Part model, mm, in its own coordinate system. A direction names the side the tool comes from. Give positions to 0.01 mm unless a question says otherwise; leave off trailing zeros. Write each loop counter-clockwise with the first axis right and the second up, starting at its lowest first coordinate (ties: lowest second). Pieces come first, ordered by that corner, then holes.
Autodesk Inventor part; units mm, degrees
ref_plane "HUELSE3_1_XY" through (11.8, 0, -12.5) normal (1, 0, 0) x (0, 0, -1)
ref_plane "HUELSE3_1_YZ" through (11.8, 0, -12.5) normal (0, 0, -1) x (0, 1, 0)
ref_plane "HUELSE3_1_ZX" through (11.8, 0, -12.5) normal (0, 1, 0) x (1, 0, 0)
sketch "Sketch_2" plane through (13, 0, 0) normal (1, 0, 0) x (0, 0, -1)
  line L0 (-29, -12) -> (-28, -13)
  line L1 (-28, -13) -> (28, -13)
  line L2 (28, -13) -> (29, -12)
  line L3 (29, -12) -> (29, 12)
  line L4 (29, 12) -> (28, 13)
  line L5 (28, 13) -> (-28, 13)
  line L6 (-28, 13) -> (-29, 12)
  line L7 (-29, 12) -> (-29, -12)
sketch "Sketch_3" plane through (0, 0, 0) normal (0, 1, 0) x (1, 0, 0)
  line L0 (13, 20.5) -> (-142, 20.5)
  line L1 (-142, 20.5) -> (-142, 24.5)
  line L2 (-142, 24.5) -> (-141, 25.5)
  line L3 (-141, 25.5) -> (13, 25.5)
  line L4 (13, 25.5) -> (13, 20.5)
  line L5 (13, 20.5) -> (-142, 20.5)
sketch "Sketch_4" plane through (0, 0, 0) normal (0, 1, 0) x (1, 0, 0)
  line L0 (13, -20.5) -> (-142, -20.5)
  line L1 (-142, -20.5) -> (-142, -16.5)
  line L2 (-142, -16.5) -> (-141, -15.5)
  line L3 (-141, -15.5) -> (13, -15.5)
  line L4 (13, -15.5) -> (13, -20.5)
  line L5 (13, -20.5) -> (-142, -20.5)
extrude "Extrusion1" add sketch "Sketch_2" against normal blind 10
sketch "Sketch_8" plane through (0, 10, 0) normal (0, 1, 0) x (1, 0, 0)
  line L0 (13, 10) -> (3, 10)
  line L1 (3, 10) -> (3, 12)
  line L2 (3, 12) -> (3.379, 11.621)
  line L3 (3.379, 11.621) -> (12.621, 11.621)
  line L4 (12.621, 11.621) -> (13, 12)
  line L5 (13, 12) -> (13, 10)
  line L6 (13, 10) -> (3, 10)
revolve "Revolution1" cut sketch "Sketch_8" angle 360 about axis through (13, 10, -10) along (-1, 0, 0)
thread "Thread1"
sketch "Sketch_9" plane through (0, 10, 0) normal (0, 1, 0) x (1, 0, 0)
  line L0 (13, -10) -> (3, -10)
  line L1 (3, -10) -> (3, -8)
  line L2 (3, -8) -> (3.379, -8.379)
  line L3 (3.379, -8.379) -> (12.621, -8.379)
  line L4 (12.621, -8.379) -> (13, -8)
  line L5 (13, -8) -> (13, -10)
  line L6 (13, -10) -> (3, -10)
revolve "Revolution2" cut sketch "Sketch_9" angle 360 about axis through (13, 10, 10) along (-1, 0, 0)
thread "Thread2"
sketch "Sketch_12" plane through (0, -10, 0) normal (0, 1, 0) x (1, 0, 0)
  line L0 (13, 10) -> (3, 10)
  line L1 (3, 10) -> (3, 12)
  line L2 (3, 12) -> (3.379, 11.621)
  line L3 (3.379, 11.621) -> (12.621, 11.621)
  line L4 (12.621, 11.621) -> (13, 12)
  line L5 (13, 12) -> (13, 10)
  line L6 (13, 10) -> (3, 10)
revolve "Revolution3" cut sketch "Sketch_12" angle 360 about axis through (13, -10, -10) along (-1, 0, 0)
thread "Thread3"
sketch "Sketch_13" plane through (0, -10, 0) normal (0, 1, 0) x (1, 0, 0)
  line L0 (13, -10) -> (3, -10)
  line L1 (3, -10) -> (3, -8)
  line L2 (3, -8) -> (3.379, -8.379)
  line L3 (3.379, -8.379) -> (12.621, -8.379)
  line L4 (12.621, -8.379) -> (13, -8)
  line L5 (13, -8) -> (13, -10)
  line L6 (13, -10) -> (3, -10)
revolve "Revolution4" cut sketch "Sketch_13" angle 360 about axis through (13, -10, 10) along (-1, 0, 0)
thread "Thread4"
sketch "Skizze_3" plane through (0, 0, 0) normal (0, 0, 1) x (1, 0, 0)
  line L0 (3, 0) -> (-117.4, 0)
  line L1 (-117.4, 0) -> (-117.4, 6)
  line L2 (-117.4, 6) -> (-111.4, 6)
  line L3 (-111.4, 6) -> (-111.4, 3)
  line L4 (-111.4, 3) -> (3, 3)
  line L5 (3, 3) -> (3, 0)
  line L6 (3, 0) -> (-117.4, 0)
revolve "Revolution5" add sketch "Skizze_3" angle 360 about axis through (3, 0, 0) along (-1, 0, 0)
sketch "Sketch_17" plane through (0, 0, 0) normal (1, 0, 0) x (0, 1, 0)
  line L0 (-10, 7.5) -> (-10, -7.5)
  line L1 (-10, -7.5) -> (10, -7.5)
  line L2 (10, -7.5) -> (10, 7.5)
  line L3 (10, 7.5) -> (-10, 7.5)
  line L4 (-5, 2.75) -> (-5, -2.75)
  line L5 (-5, -2.75) -> (5, -2.75)
  line L6 (5, -2.75) -> (5, 2.75)
  line L7 (5, 2.75) -> (-5, 2.75)
extrude "Extrusion2" cut sketch "Sketch_17" along normal blind 3
sketch "Sketch10" plane through (13, 0, 0) normal (1, 0, 0) x (0, 0, -1)
  point P0 (12.5, 0)
hole "Hole1" at (13, 0, -12.5) direction (-1, 0, 0) diameter 5 depth 1.2 tip angle 120
sketch "Sketch11" plane through (13, 0, 0) normal (1, 0, 0) x (0, 0, -1)
  point P0 (-12.5, 0)
hole "Hole2" at (13, 0, 12.5) direction (-1, 0, 0) diameter 5 depth 1.2 tip angle 120
sketch "Sketch12" plane through (13, 13, 28) normal (0, 1, 0) x (1, 0, 0)
  point P0 (-5, 48.5)
hole "Hole3" at (8, 13, -20.5) direction (0, -1, 0) diameter 3.242 depth 13 countersink diameter 4 countersink angle 90
sketch "Sketch13" plane through (13, 13, 28) normal (0, 1, 0) x (1, 0, 0)
  point P0 (-5, 7.5)
hole "Hole4" at (8, 13, 20.5) direction (0, -1, 0) diameter 3.242 depth 13 countersink diameter 4 countersink angle 90
revolve "Revolution6" add sketch "Sketch_4" angle 360 about axis through (13, 0, 20.5) along (1, 0, 0)
revolve "Revolution7" add sketch "Sketch_3" angle 360 about axis through (13, 0, -20.5) along (1, 0, 0)
sketch "Sketch_20" plane through (13, 0, 0) normal (1, 0, 0) x (0, 0, -1)
  arc A0 (-1.6342, -0.5011) -> (-1.2511, -1.1647) centre (-1.364, -0.7875) ccw
  arc A1 (-0.3831, -1.6659) -> (-1.2511, -1.1647) centre (-1.0536, -1.8249) ccw
  arc A2 (-0.3831, -1.6659) -> (0.3831, -1.6659) centre (0, -1.575) ccw
  arc A3 (1.2511, -1.1647) -> (0.3831, -1.6659) centre (1.0536, -1.8249) ccw
  arc A4 (1.2511, -1.1647) -> (1.6342, -0.5011) centre (1.364, -0.7875) ccw
  arc A5 (1.6342, 0.5011) -> (1.6342, -0.5011) centre (2.1072, 0) ccw
  arc A6 (1.6342, 0.5011) -> (1.2511, 1.1647) centre (1.364, 0.7875) ccw
  arc A7 (0.3831, 1.6659) -> (1.2511, 1.1647) centre (1.0536, 1.8249) ccw
  arc A8 (0.3831, 1.6659) -> (-0.3831, 1.6659) centre (0, 1.575) ccw
  arc A9 (-1.2511, 1.1647) -> (-0.3831, 1.6659) centre (-1.0536, 1.8249) ccw
  arc A10 (-1.2511, 1.1647) -> (-1.6342, 0.5011) centre (-1.364, 0.7875) ccw
  arc A11 (-1.6342, -0.5011) -> (-1.6342, 0.5011) centre (-2.1072, 0) ccw
extrude "Extrusion3" cut sketch "Sketch_20" against normal blind 2
sketch "Pattern_2_SKETCH_1" plane through (13, 0, 0) normal (1, 0, 0) x (0, 0, -1)
  arc A0 (18.8658, -0.5011) -> (19.2489, -1.1647) centre (19.136, -0.7875) ccw
  arc A1 (20.1169, -1.6659) -> (19.2489, -1.1647) centre (19.4464, -1.8249) ccw
  arc A2 (20.1169, -1.6659) -> (20.8831, -1.6659) centre (20.5, -1.575) ccw
  arc A3 (21.7511, -1.1647) -> (20.8831, -1.6659) centre (21.5536, -1.8249) ccw
  arc A4 (21.7511, -1.1647) -> (22.1342, -0.5011) centre (21.864, -0.7875) ccw
  arc A5 (22.1342, 0.5011) -> (22.1342, -0.5011) centre (22.6072, 0) ccw
  arc A6 (22.1342, 0.5011) -> (21.7511, 1.1647) centre (21.864, 0.7875) ccw
  arc A7 (20.8831, 1.6659) -> (21.7511, 1.1647) centre (21.5536, 1.8249) ccw
  arc A8 (20.8831, 1.6659) -> (20.1169, 1.6659) centre (20.5, 1.575) ccw
  arc A9 (19.2489, 1.1647) -> (20.1169, 1.6659) centre (19.4464, 1.8249) ccw
  arc A10 (19.2489, 1.1647) -> (18.8658, 0.5011) centre (19.136, 0.7875) ccw
  arc A11 (18.8658, -0.5011) -> (18.8658, 0.5011) centre (18.3928, 0) ccw
sketch "Pattern_2_SKETCH_2" plane through (13, 0, 0) normal (1, 0, 0) x (0, 0, -1)
  arc A0 (-22.1342, -0.5011) -> (-21.7511, -1.1647) centre (-21.864, -0.7875) ccw
  arc A1 (-20.8831, -1.6659) -> (-21.7511, -1.1647) centre (-21.5536, -1.8249) ccw
  arc A2 (-20.8831, -1.6659) -> (-20.1169, -1.6659) centre (-20.5, -1.575) ccw
  arc A3 (-19.2489, -1.1647) -> (-20.1169, -1.6659) centre (-19.4464, -1.8249) ccw
  arc A4 (-19.2489, -1.1647) -> (-18.8658, -0.5011) centre (-19.136, -0.7875) ccw
  arc A5 (-18.8658, 0.5011) -> (-18.8658, -0.5011) centre (-18.3928, 0) ccw
  arc A6 (-18.8658, 0.5011) -> (-19.2489, 1.1647) centre (-19.136, 0.7875) ccw
  arc A7 (-20.1169, 1.6659) -> (-19.2489, 1.1647) centre (-19.4464, 1.8249) ccw
  arc A8 (-20.1169, 1.6659) -> (-20.8831, 1.6659) centre (-20.5, 1.575) ccw
  arc A9 (-21.7511, 1.1647) -> (-20.8831, 1.6659) centre (-21.5536, 1.8249) ccw
  arc A10 (-21.7511, 1.1647) -> (-22.1342, 0.5011) centre (-21.864, 0.7875) ccw
  arc A11 (-22.1342, -0.5011) -> (-22.1342, 0.5011) centre (-22.6072, 0) ccw
extrude "Extrusion4" cut sketch "Pattern_2_SKETCH_1" against normal blind 2
extrude "Extrusion5" cut sketch "Pattern_2_SKETCH_2" against normal blind 2
sketch "Sketch_22" plane through (0, 0, 0) normal (0, 1, 0) x (1, 0, 0)
  line L0 (13, 0) -> (12.6, 0)
  line L1 (12.6, 0) -> (12.6, 3)
  arc A0 (12.6, 3) -> (12.1, 3.5) centre (12.1, 3) ccw
  line L2 (12.1, 3.5) -> (9.5, 3.5)
  line L3 (9.5, 3.5) -> (9.5, 4)
  line L4 (9.5, 4) -> (13, 4)
  line L5 (13, 4) -> (13, 0)
  line L6 (13, 0) -> (12.6, 0)
revolve "Revolution8" cut sketch "Sketch_22" angle 360 about axis through (13, 0, 0) along (-1, 0, 0)
sketch "Pattern_3_SKETCH_1" plane through (0, 0, 20.5) normal (0, 1, 0) x (1, 0, 0)
  line L0 (13, 0) -> (12.6, 0)
  line L1 (12.6, 0) -> (12.6, 3)
  arc A0 (12.6, 3) -> (12.1, 3.5) centre (12.1, 3) ccw
  line L2 (12.1, 3.5) -> (9.5, 3.5)
  line L3 (9.5, 3.5) -> (9.5, 4)
  line L4 (9.5, 4) -> (13, 4)
  line L5 (13, 4) -> (13, 0)
  line L6 (13, 0) -> (12.6, 0)
sketch "Pattern_3_SKETCH_2" plane through (0, 0, -20.5) normal (0, 1, 0) x (1, 0, 0)
  line L0 (13, 0) -> (12.6, 0)
  line L1 (12.6, 0) -> (12.6, 3)
  arc A0 (12.6, 3) -> (12.1, 3.5) centre (12.1, 3) ccw
  line L2 (12.1, 3.5) -> (9.5, 3.5)
  line L3 (9.5, 3.5) -> (9.5, 4)
  line L4 (9.5, 4) -> (13, 4)
  line L5 (13, 4) -> (13, 0)
  line L6 (13, 0) -> (12.6, 0)
revolve "Revolution9" cut sketch "Pattern_3_SKETCH_1" angle 360 about axis through (13, 0, 20.5) along (-1, 0, 0)
revolve "Revolution10" cut sketch "Pattern_3_SKETCH_2" angle 360 about axis through (13, 0, -20.5) along (-1, 0, 0)
ref_plane "HUELSE3_1_XY" through (11.8, 0, -12.5) normal (1, 0, 0) x (0, 0, -1)
ref_plane "HUELSE3_1_YZ" through (11.8, 0, -12.5) normal (0, 0, -1) x (0, 1, 0)
ref_plane "HUELSE3_1_ZX" through (11.8, 0, -12.5) normal (0, 1, 0) x (1, 0, 0)
ref_plane "HUELSE3_2_XY" through (11.8, 0, 12.5) normal (1, 0, 0) x (0, 0, -1)
ref_plane "HUELSE3_2_YZ" through (11.8, 0, 12.5) normal (0, 0, -1) x (0, 1, 0)
ref_plane "HUELSE3_2_ZX" through (11.8, 0, 12.5) normal (0, 1, 0) x (1, 0, 0)
ref_plane "dfm_k_XY" through (0, 0, 0) normal (-1, 0, 0) x (0, 0, -1)
ref_plane "dfm_k_YZ" through (0, 0, 0) normal (0, 0, -1) x (0, -1, 0)
ref_plane "dfm_k_ZX" through (0, 0, 0) normal (0, -1, 0) x (-1, 0, 0)
properties part number "170831 DFM-12-100-P-A-GF---(K)"
1) Two-plate mould, pull along Z, no slides. Class faces 5 (the face through (-111.4, -3, 1)), 6 (the face through (8.06, 11.1, 11.19)), 7 (the face through (8, 13, 0)): +Z half, -Z half, draft (parallel to the pull), parting line (faces both ways), or undercut.
Answers follow:
face 5: undercut
face 6: undercut
face 7: draft
2) 3-axis set-ups, long thin cutter, end or side, ignore diameter. For faces 1 (the face through (8, -13, 0)), 2 (the face through (7.513, 8.62, -18.954)), 3 (the face through (12.6, -1.4, -1.3)), 4 (the face through (-67.992, 0.22, 25.495)): which of +Z, -Z, +X, -X, +Y, -Y reach the whole face in a straight line?
Answers follow:
face 1: +Z, -Z, +X, -X, -Y
face 2: +Y
face 3: +X
face 4: -X
3) Saw through at A-A, the plane y = -10. Write the cut outline in (x, z), then the cut area to 3 significant figures.
Answers follow:
outline: (3, -29) - (13, -29) - (13, -12) - (12.62, -11.62) - (3.38, -11.62) - (3, -12) - close; (3, -8) - (3.38, -8.38) - (12.62, -8.38) - (13, -8) - (13, 8) - (12.62, 8.38) - (3.38, 8.38) - (3, 8) - close; (3, 12) - (3.38, 11.62) - (12.62, 11.62) - (13, 12) - (13, 29) - (3, 29) - close
area: 515 mm2
4) Saw through at B-B, the plane x = 8. Write the cut outline in (y, z), then the cut area to 3 significant figures.
Answers follow:
outline: (-13, -28) - (-12, -29) - (12, -29) - (13, -28) - (13, -22.5) - (12.62, -22.12) - (4.73, -22.12) arc R5 ccw to (4.73, -18.88) - (12.62, -18.88) - (13, -18.5) - (13, 18.5) - (12.62, 18.88) - (4.73, 18.88) arc R5 ccw to (4.73, 22.12) - (12.62, 22.12) - (13, 22.5) - (13, 28) - (12, 29) - (-12, 29) - (-13, 28) - close; hole circle Ø3.24 at (-10, -10); hole circle Ø3.24 at (-10, 10); hole circle Ø3.24 at (10, -10); hole circle Ø3.24 at (10, 10)
area: 1,420 mm2
5) Pin check, flat tips, straight feed: pin 1 Ø1 at (y, z) = (1, -15.5) entering from -X; pin 2 Ø9.5 at (y, z) = (2.5, 3) entering from -X; pin 3 Ø1.5 at (y, z) = (-0.5, 18) entering from +X; pin 4 Ø1.9 at (y, z) = (-10, -10) entering from +X. Stop position of each tip, or through.
Answers follow:
pin 1: stops at x = -141.4
pin 2: stops at x = -117.4
pin 3: stops at x = 12.6
pin 4: passes through
6) Wall check: L1, parallel to Y at x = 5.25, z = 10; L2, parallel to Z at x = 5.75, y = -10; L3, parallel to Z at x = 12.8, y = 0. Give the ranges that are in metal, low to high.
Answers follow:
L1: y = -13 to -11.62, -8.38 to 8.38, 11.62 to 13
L2: z = -29 to -11.62, -8.38 to 8.38, 11.62 to 29
L3: z = -29 to -24.5, -16.5 to -15, -10 to -4, 4 to 10, 15 to 16.5, 24.5 to 29
